The listing builds one solid part. Answer for the finished solid, in the listing's coordinates (mm). A direction names the side the tool comes from. Round coordinates to 2 decimals unless told otherwise and drop trailing zeros. Write each loop counter-clockwise with the first axis right and the second up, starting at its lowest first coordinate (ties: lowest second). Pieces come first, ordered by that corner, then holes. Notation, with made-up numbers: (70.5, -15) - (86.5, -15) arc R12 ccw to (86.5, 4) - close; hole circle Ø4 at (61, 79). An arc over 180 degrees is marked (long way). Answer as CSV lines item,"result". Start each with the question number.
Item 1: Straight lines are drawn through the part: line 1 along Z through (x, y) = (4, -5); line 2 along Z through (x, y) = (6, -1.5); line 3 along X through (y, z) = (-7.75, -15). For each, find the intervals that lie inside material, in ascending order. Write a range as [from, to].
Item 2: Flat-ended cylindrical pins translate along their axes: pin 1 (1 mm diameter, centred on x = 18, y = -2, fed in from +Z); pin 2 (0.8 mm diameter, centred on y = -6.5, z = -14, fed in from +X); pin 3 (5 mm diameter, centred on y = -7, z = 12, fed in from -X). Find the tip coordinate at first contact, or state that the pin passes through.
Item 3: For a pull along X with two mould halves and no side action, classify faces 5 (the cylindrical face through (6.6, -3.5, 12.4)), 6 (the flat face through (3.85, -2, 20)), 7 (the flat face through (9.35, -2, -10)), 8 (the flat face through (43, -8, 30.905)) as pulls with the +X half, pulls with the -X half, needs draft (parallel to the pull), parting line crosses it, or undercut.
Item 4: A cutting plane is placed at B-B on z = 15.1. Determine the outline of the cut face in (x, y), and give its area (3 significant figures).
Item 5: A cutting plane is placed at A-A on x = 13. Determine the outline of the cut face in (y, z), and give its area (3 significant figures).
Item 6: A cutting plane is placed at C-C on y = -0.75. State how many separate pieces and enclosed holes the cut face has, and give its area (3 significant figures).
Item 7: A cutting plane is placed at D-D on x = 6.6. Determine the outline of the cut face in (y, z), and give its area (3 significant figures).
Item 8: Which of the six approach directions +Z, -Z, +X, -X, +Y, -Y give full straight-line access (tool end or side, diameter ignored) to faces 1 (the cylindrical face through (-6.685, -7.564, -21.251)), 2 (the flat face through (8, -3, -18.8)), 3 (the cylindrical face through (38.57, -7.564, 30.304)), 4 (the cylindrical face through (47.685, -7.564, 21.251))?
```python
from build123d import *

# Parameters (mm, degrees)
BOSS_EXTRUDE1_DEPTH = 41
BOSS_EXTRUDE2_REACH = 50.098
SKETCH2_R           = 1
SKETCH4_W           = 5.5
SKETCH4_H           = 13.1
SKETCH4_R           = 1
CUT_EXTRUDE1_DEPTH  = 7
SKETCH5_R           = 2.25
BOSS_EXTRUDE3_DEPTH = 2
BOSS_EXTRUDE4_REACH = 59.938
SKETCH6_W           = 5.5
SKETCH6_H           = 2.85


with BuildPart() as part:
    # Sketch1 → Boss-Extrude1 (new body)
    with BuildSketch(Plane(origin=(0, 0, 0), x_dir=(0, 0, -1), z_dir=(1, 0, 0))):
        with BuildLine():
            Line((-8.55, 0), (-6.55, 0))
            ThreePointArc((-6.55, 0), (0, -6.55), (6.55, 0))
            Line((6.55, 0), (8.55, 0))
            ThreePointArc((8.55, 0), (15.1, -6.55), (21.65, 0))
            Line((21.65, 0), (23.65, 0))
            Line((23.65, 0), (23.65, -8.55))
            Line((23.65, -8.55), (-23.65, -8.55))
            Line((-23.65, -8.55), (-23.65, 0))
            Line((-23.65, 0), (-21.65, 0))
            ThreePointArc((-21.65, 0), (-15.1, -6.55), (-8.55, 0))
        make_face()
    extrude(amount=BOSS_EXTRUDE1_DEPTH)

    # Sketch2 → Boss-Extrude2 (add, up to next)
    with BuildSketch(Plane(origin=(0, 0, 0), x_dir=(1, 0, 0), z_dir=(0, 1, 0)), mode=Mode.PRIVATE) as boss_extrude2_sk1:
        with Locations(Location((6.6, 3.7, 0), (0, 0, 270))):
            Circle(SKETCH2_R)
    boss_extrude2_tool1 = extrude(boss_extrude2_sk1.sketch, amount=-BOSS_EXTRUDE2_REACH, mode=Mode.PRIVATE) - part.part
    # Sketch2 → Boss-Extrude2 (add, up to next)
    with BuildSketch(Plane(origin=(0, 0, 0), x_dir=(1, 0, 0), z_dir=(0, 1, 0)), mode=Mode.PRIVATE) as boss_extrude2_sk2:
        with Locations(Location((6.6, -3.7, 0), (0, 0, 270))):
            Circle(SKETCH2_R)
    boss_extrude2_tool2 = extrude(boss_extrude2_sk2.sketch, amount=-BOSS_EXTRUDE2_REACH, mode=Mode.PRIVATE) - part.part
    # Sketch2 → Boss-Extrude2 (add, up to next)
    with BuildSketch(Plane(origin=(0, 0, 0), x_dir=(1, 0, 0), z_dir=(0, 1, 0)), mode=Mode.PRIVATE) as boss_extrude2_sk3:
        with Locations(Location((6.6, -11.4, 0), (0, 0, 270))):
            Circle(SKETCH2_R)
    boss_extrude2_tool3 = extrude(boss_extrude2_sk3.sketch, amount=-BOSS_EXTRUDE2_REACH, mode=Mode.PRIVATE) - part.part
    # Sketch2 → Boss-Extrude2 (add, up to next)
    with BuildSketch(Plane(origin=(0, 0, 0), x_dir=(1, 0, 0), z_dir=(0, 1, 0)), mode=Mode.PRIVATE) as boss_extrude2_sk4:
        with Locations(Location((6.6, -18.8, 0), (0, 0, 270))):
            Circle(SKETCH2_R)
    boss_extrude2_tool4 = extrude(boss_extrude2_sk4.sketch, amount=-BOSS_EXTRUDE2_REACH, mode=Mode.PRIVATE) - part.part
    # Sketch2 → Boss-Extrude2 (add, up to next)
    with BuildSketch(Plane(origin=(0, 0, 0), x_dir=(1, 0, 0), z_dir=(0, 1, 0)), mode=Mode.PRIVATE) as boss_extrude2_sk5:
        with Locations(Location((6.6, 18.8, 0), (0, 0, 270))):
            Circle(SKETCH2_R)
    boss_extrude2_tool5 = extrude(boss_extrude2_sk5.sketch, amount=-BOSS_EXTRUDE2_REACH, mode=Mode.PRIVATE) - part.part
    # Sketch2 → Boss-Extrude2 (add, up to next)
    with BuildSketch(Plane(origin=(0, 0, 0), x_dir=(1, 0, 0), z_dir=(0, 1, 0)), mode=Mode.PRIVATE) as boss_extrude2_sk6:
        with Locations(Location((6.6, 11.4, 0), (0, 0, 270))):
            Circle(SKETCH2_R)
    boss_extrude2_tool6 = extrude(boss_extrude2_sk6.sketch, amount=-BOSS_EXTRUDE2_REACH, mode=Mode.PRIVATE) - part.part
    add(boss_extrude2_tool1.solids().sort_by_distance((6.6, 0, -3.7))[0])
    add(boss_extrude2_tool2.solids().sort_by_distance((6.6, 0, 3.7))[0])
    add(boss_extrude2_tool3.solids().sort_by_distance((6.6, 0, 11.4))[0])
    add(boss_extrude2_tool4.solids().sort_by_distance((6.6, 0, 18.8))[0])
    add(boss_extrude2_tool5.solids().sort_by_distance((6.6, 0, -18.8))[0])
    add(boss_extrude2_tool6.solids().sort_by_distance((6.6, 0, -11.4))[0])

    # Sketch4 → Cut-Extrude1 (cut)
    # profile 1 of 3: a face of its own
    with BuildSketch(Plane(origin=(0, 0, 0), x_dir=(1, 0, 0), z_dir=(0, 1, 0))):
        with Locations((6.6, 0)):
            Rectangle(SKETCH4_W, SKETCH4_H)
        with Locations(Location((6.6, 3.7, 0), (0, 0, 270))):
            Circle(SKETCH4_R, mode=Mode.SUBTRACT)
        with Locations(Location((6.6, -3.7, 0), (0, 0, 270))):
            Circle(SKETCH4_R, mode=Mode.SUBTRACT)
    # profile 2 of 3: a face of its own
    with BuildSketch(Plane(origin=(0, 0, 0), x_dir=(1, 0, 0), z_dir=(0, 1, 0))):
        with Locations((6.6, -15.1)):
            Rectangle(SKETCH4_W, SKETCH4_H)
        with Locations(Location((6.6, -11.4, 0), (0, 0, 90))):
            Circle(SKETCH4_R, mode=Mode.SUBTRACT)
        with Locations(Location((6.6, -18.8, 0), (0, 0, 90))):
            Circle(SKETCH4_R, mode=Mode.SUBTRACT)
    # profile 3 of 3: a face of its own
    with BuildSketch(Plane(origin=(0, 0, 0), x_dir=(1, 0, 0), z_dir=(0, 1, 0))):
        with Locations((6.6, 15.1)):
            Rectangle(SKETCH4_W, SKETCH4_H)
        with Locations(Location((6.6, 11.4, 0), (0, 0, 90))):
            Circle(SKETCH4_R, mode=Mode.SUBTRACT)
        with Locations(Location((6.6, 18.8, 0), (0, 0, 90))):
            Circle(SKETCH4_R, mode=Mode.SUBTRACT)
    extrude(amount=-CUT_EXTRUDE1_DEPTH, mode=Mode.SUBTRACT)

    # Sketch5 → Boss-Extrude3 (add)
    # profile 1 of 4: a face of its own
    with BuildSketch(Plane.XZ.offset(8.55)):
        with BuildLine():
            Line((0, 23.65), (0, 20.65))
            Line((0, 20.65), (-5.25520382, 20.65))
            ThreePointArc((-5.25520382, 20.65), (-6.669417382, 21.235786438), (-7.25520382, 22.65))
            Line((-7.25520382, 22.65), (-7.25520382, 28.90520382))
            ThreePointArc((-7.25520382, 28.90520382), (-6.669417382, 30.319417382), (-5.25520382, 30.90520382))
            Line((-5.25520382, 30.90520382), (1, 30.90520382))
            ThreePointArc((1, 30.90520382), (2.414213562, 30.319417382), (3, 28.90520382))
            Line((3, 28.90520382), (3, 23.65))
            Line((3, 23.65), (0, 23.65))
        make_face()
        with Locations(Location((-3.00520382, 26.65520382, 0), (0, 0, 270))):
            Circle(SKETCH5_R, mode=Mode.SUBTRACT)
    # profile 2 of 4: a face of its own
    with BuildSketch(Plane.XZ.offset(8.55)):
        with BuildLine():
            Line((0, -23.65), (3, -23.65))
            Line((3, -23.65), (3, -28.90520382))
            ThreePointArc((3, -28.90520382), (2.414213562, -30.319417382), (1, -30.90520382))
            Line((1, -30.90520382), (-5.25520382, -30.90520382))
            ThreePointArc((-5.25520382, -30.90520382), (-6.669417382, -30.319417382), (-7.25520382, -28.90520382))
            Line((-7.25520382, -28.90520382), (-7.25520382, -22.65))
            ThreePointArc((-7.25520382, -22.65), (-6.669417382, -21.235786438), (-5.25520382, -20.65))
            Line((-5.25520382, -20.65), (0, -20.65))
            Line((0, -20.65), (0, -23.65))
        make_face()
        with Locations(Location((-3.00520382, -26.65520382, 0), (0, 0, 90))):
            Circle(SKETCH5_R, mode=Mode.SUBTRACT)
    # profile 3 of 4: a face of its own
    with BuildSketch(Plane.XZ.offset(8.55)):
        with BuildLine():
            Line((41, -23.65), (41, -20.65))
            Line((41, -20.65), (46.25520382, -20.65))
            ThreePointArc((46.25520382, -20.65), (47.669417382, -21.235786438), (48.25520382, -22.65))
            Line((48.25520382, -22.65), (48.25520382, -28.90520382))
            ThreePointArc((48.25520382, -28.90520382), (47.669417382, -30.319417382), (46.25520382, -30.90520382))
            Line((46.25520382, -30.90520382), (40, -30.90520382))
            ThreePointArc((40, -30.90520382), (38.585786438, -30.319417382), (38, -28.90520382))
            Line((38, -28.90520382), (38, -23.65))
            Line((38, -23.65), (41, -23.65))
        make_face()
        with Locations(Location((44.00520382, -26.65520382, 0), (0, 0, 270))):
            Circle(SKETCH5_R, mode=Mode.SUBTRACT)
    # profile 4 of 4: a face of its own
    with BuildSketch(Plane.XZ.offset(8.55)):
        with BuildLine():
            Line((41, 23.65), (38, 23.65))
            Line((38, 23.65), (38, 28.90520382))
            ThreePointArc((38, 28.90520382), (38.585786438, 30.319417382), (40, 30.90520382))
            Line((40, 30.90520382), (46.25520382, 30.90520382))
            ThreePointArc((46.25520382, 30.90520382), (47.669417382, 30.319417382), (48.25520382, 28.90520382))
            Line((48.25520382, 28.90520382), (48.25520382, 22.65))
            ThreePointArc((48.25520382, 22.65), (47.669417382, 21.235786438), (46.25520382, 20.65))
            Line((46.25520382, 20.65), (41, 20.65))
            Line((41, 20.65), (41, 23.65))
        make_face()
        with Locations(Location((44.00520382, 26.65520382, 0), (0, 0, 90))):
            Circle(SKETCH5_R, mode=Mode.SUBTRACT)
    extrude(amount=-BOSS_EXTRUDE3_DEPTH)

    # Boss-Extrude4: up to this face of the body (flat: up to its plane)
    boss_extrude4_end = Plane(part.part.faces().sort_by_distance((6.6, -7, -15.1))[0])
    # Sketch6 → Boss-Extrude4 (add, up to the picked face)
    with BuildSketch(Plane(origin=(0, 0, 0), x_dir=(1, 0, 0), z_dir=(0, 1, 0)), mode=Mode.PRIVATE) as boss_extrude4_sk1:
        with Locations((6.6, -5.125)):
            Rectangle(SKETCH6_W, SKETCH6_H)
    boss_extrude4_tool1 = split(extrude(boss_extrude4_sk1.sketch, amount=-BOSS_EXTRUDE4_REACH, mode=Mode.PRIVATE), bisect_by=boss_extrude4_end, keep=Keep.BOTH, mode=Mode.PRIVATE)
    # Sketch6 → Boss-Extrude4 (add, up to the picked face)
    with BuildSketch(Plane(origin=(0, 0, 0), x_dir=(1, 0, 0), z_dir=(0, 1, 0)), mode=Mode.PRIVATE) as boss_extrude4_sk2:
        with Locations((6.6, 5.125)):
            Rectangle(SKETCH6_W, SKETCH6_H)
    boss_extrude4_tool2 = split(extrude(boss_extrude4_sk2.sketch, amount=-BOSS_EXTRUDE4_REACH, mode=Mode.PRIVATE), bisect_by=boss_extrude4_end, keep=Keep.BOTH, mode=Mode.PRIVATE)
    # Sketch6 → Boss-Extrude4 (add, up to the picked face)
    with BuildSketch(Plane(origin=(0, 0, 0), x_dir=(1, 0, 0), z_dir=(0, 1, 0)), mode=Mode.PRIVATE) as boss_extrude4_sk3:
        with Locations((6.6, -20.225)):
            Rectangle(SKETCH6_W, SKETCH6_H)
    boss_extrude4_tool3 = split(extrude(boss_extrude4_sk3.sketch, amount=-BOSS_EXTRUDE4_REACH, mode=Mode.PRIVATE), bisect_by=boss_extrude4_end, keep=Keep.BOTH, mode=Mode.PRIVATE)
    # Sketch6 → Boss-Extrude4 (add, up to the picked face)
    with BuildSketch(Plane(origin=(0, 0, 0), x_dir=(1, 0, 0), z_dir=(0, 1, 0)), mode=Mode.PRIVATE) as boss_extrude4_sk4:
        with Locations((6.6, -9.975)):
            Rectangle(SKETCH6_W, SKETCH6_H)
    boss_extrude4_tool4 = split(extrude(boss_extrude4_sk4.sketch, amount=-BOSS_EXTRUDE4_REACH, mode=Mode.PRIVATE), bisect_by=boss_extrude4_end, keep=Keep.BOTH, mode=Mode.PRIVATE)
    # Sketch6 → Boss-Extrude4 (add, up to the picked face)
    with BuildSketch(Plane(origin=(0, 0, 0), x_dir=(1, 0, 0), z_dir=(0, 1, 0)), mode=Mode.PRIVATE) as boss_extrude4_sk5:
        with Locations((6.6, 9.975)):
            Rectangle(SKETCH6_W, SKETCH6_H)
    boss_extrude4_tool5 = split(extrude(boss_extrude4_sk5.sketch, amount=-BOSS_EXTRUDE4_REACH, mode=Mode.PRIVATE), bisect_by=boss_extrude4_end, keep=Keep.BOTH, mode=Mode.PRIVATE)
    # Sketch6 → Boss-Extrude4 (add, up to the picked face)
    with BuildSketch(Plane(origin=(0, 0, 0), x_dir=(1, 0, 0), z_dir=(0, 1, 0)), mode=Mode.PRIVATE) as boss_extrude4_sk6:
        with Locations((6.6, 20.225)):
            Rectangle(SKETCH6_W, SKETCH6_H)
    boss_extrude4_tool6 = split(extrude(boss_extrude4_sk6.sketch, amount=-BOSS_EXTRUDE4_REACH, mode=Mode.PRIVATE), bisect_by=boss_extrude4_end, keep=Keep.BOTH, mode=Mode.PRIVATE)
    add(boss_extrude4_tool1.solids().sort_by(Axis((6.6, 0, 5.125), (0, -1, 0)))[0])
    add(boss_extrude4_tool2.solids().sort_by(Axis((6.6, 0, -5.125), (0, -1, 0)))[0])
    add(boss_extrude4_tool3.solids().sort_by(Axis((6.6, 0, 20.225), (0, -1, 0)))[0])
    add(boss_extrude4_tool4.solids().sort_by(Axis((6.6, 0, 9.975), (0, -1, 0)))[0])
    add(boss_extrude4_tool5.solids().sort_by(Axis((6.6, 0, -9.975), (0, -1, 0)))[0])
    add(boss_extrude4_tool6.solids().sort_by(Axis((6.6, 0, -20.225), (0, -1, 0)))[0])


solid = part.part
```
Geometry says:
1,line 1,"z = [-23.65, -18.8], [-11.4, -3.7], [3.7, 11.4], [18.8, 23.65]"
1,line 2,"z = [-23.65, -18], [-12.2, -2.9], [2.9, 12.2], [18, 23.65]"
1,line 3,"x = [0, 41]"
2,pin 1,"stops at z = 23.65"
2,pin 2,"stops at x = 41"
2,pin 3,"stops at x = 0"
3,face 5,"undercut"
3,face 6,"pulls with the -X half"
3,face 7,"pulls with the +X half"
3,face 8,"needs draft"
4,outline,"(0, -8.55) - (41, -8.55) - (41, -6.55) - (9.35, -6.55) - (9.35, -7) - (3.85, -7) - (3.85, -6.55) - (0, -6.55) - close"
4,area,"79.5 mm^2"
5,outline,"(-8.55, -23.65) - (0, -23.65) - (0, -21.65) arc R6.55 cw to (0, -8.55) - (0, -6.55) arc R6.55 cw to (0, 6.55) - (0, 8.55) arc R6.55 cw to (0, 21.65) - (0, 23.65) - (-8.55, 23.65) - close"
5,area,"202 mm^2"
6,separate pieces,"4"
6,enclosed holes,"0"
6,area,"441 mm^2"
7,outline,"(-8.55, -23.65) - (0, -23.65) - (0, -17.8) - (-7, -17.8) - (-7, -12.4) - (0, -12.4) - (0, -2.7) - (-7, -2.7) - (-7, 2.7) - (0, 2.7) - (0, 12.4) - (-7, 12.4) - (-7, 17.8) - (0, 17.8) - (0, 23.65) - (-8.55, 23.65) - close"
7,area,"291 mm^2"
8,face 1,"-X, +Y, -Y"
8,face 2,"+Y"
8,face 3,"+Z, +Y, -Y"
8,face 4,"+X, +Y, -Y"
